from build123d import *

# Parameters (mm, degrees)
SKETCH1_W               = 40
SKETCH1_H               = 9
BOSS_EXTRUDE1_DEPTH     = 7
CUT_EXTRUDE1_DEPTH      = 5
CUT_EXTRUDE1_DEPTH_BACK = 10
SKETCH2_R               = 1
SKETCH2_R_2             = 1.4
FILLET1_R               = 10
FILLET2_R               = 0.5
SKETCH3_R               = 1.75
CUT_EXTRUDE6_DEPTH      = 3.8
SKETCH4_W               = 3.5
SKETCH4_H               = 0.5
CUT_EXTRUDE7_DEPTH      = 2.5


with BuildPart() as part:
    # Sketch1 → Boss-Extrude1 (new body)
    with BuildSketch(Plane(origin=(0, 0, 0), x_dir=(1, 0, 0), z_dir=(0, 1, 0))):
        with Locations((20, 4.5)):
            Rectangle(SKETCH1_W, SKETCH1_H)
    extrude(amount=BOSS_EXTRUDE1_DEPTH)

    # Sketch2 → Cut-Extrude1 (cut, two sides: drawn at the far end of the back side and taken through both)
    with BuildSketch(Plane(origin=(0, 7, 0), x_dir=(1, 0, 0), z_dir=(0, 1, 0)).offset(-CUT_EXTRUDE1_DEPTH_BACK)):
        with Locations(Location((8, 4, 0), (0, 0, 90))):
            Circle(SKETCH2_R)
        with Locations(Location((32, 4, 0), (0, 0, 90))):
            Circle(SKETCH2_R)
        with Locations(Location((20, 4, 0), (0, 0, 90))):
            Circle(SKETCH2_R_2)
        with BuildLine():
            ThreePointArc((21.734935157, 2.2), (20, 1.5), (18.265064843, 2.2))
            Line((18.265064843, 2.2), (11, 2.2))
            Line((11, 2.2), (16, 0.75))
            Line((16, 0.75), (24, 0.75))
            Line((24, 0.75), (29, 2.2))
            Line((29, 2.2), (21.734935157, 2.2))
        make_face()
        Polygon((13, 0.75), (8, 2.2), (3, 0.75), align=None)
        Polygon((37, 0.75), (32, 2.2), (27, 0.75), align=None)
        Polygon((0, 0.75), (5, 2.2), (0, 2.2), align=None)
        Polygon((40, 2.2), (35, 2.2), (40, 0.75), align=None)
    extrude(amount=CUT_EXTRUDE1_DEPTH + CUT_EXTRUDE1_DEPTH_BACK, mode=Mode.SUBTRACT)

    # Fillet1
    fillet1_edges = [part.edges().sort_by_distance(p)[0] for p in [
        (32, 3.5, -2.2),
        (8, 3.5, -2.2),
    ]]
    fillet(fillet1_edges, radius=FILLET1_R)

    # Fillet2
    # the kernel refuses this fillet: 0.5 mm, written as the material it adds along each edge
    with BuildSketch(Plane(origin=(24, 7, -0.75), x_dir=(0.9604291387787307, 0, -0.27852445024583705), z_dir=(0, -1, 0))) as fillet2_piece_1:
        with BuildLine():
            CenterArc((FILLET2_R * 0.142073204655, -FILLET2_R), FILLET2_R, 90, 16.172159016)
            Line((-FILLET2_R * 0.136451245591, -FILLET2_R * 0.0395708612213), (0, 0))
            Line((0, 0), (FILLET2_R * 0.142073204655, 0))
        make_face()
    extrude(amount=7)
    with BuildSketch(Plane(origin=(16, 0, -0.75), x_dir=(1, 0, 0), z_dir=(0, 1, 0))) as fillet2_piece_2:
        with BuildLine():
            CenterArc((FILLET2_R * 0.142073204655, FILLET2_R), FILLET2_R, 253.827840984, 16.172159016)
            Line((-FILLET2_R * 0.136451245591, FILLET2_R * 0.0395708612213), (0, 0))
            Line((0, 0), (FILLET2_R * 0.142073204655, 0))
        make_face()
    extrude(amount=7)
    # the kernel refuses this fillet: 0.5 mm, written as the material it takes off along each edge
    with BuildSketch(Plane(origin=(0, 7.939001537, -0.75), x_dir=(0.960429138778732, 0, -0.2785244502458324), z_dir=(0, -1, 0)), Plane(origin=(40, 7.939001537, -0.75), x_dir=(0, 0, 1), z_dir=(0, -1, 0))) as fillet2_2_piece_1:
        with BuildLine():
            CenterArc((FILLET2_R * 0.75120122935, FILLET2_R), FILLET2_R, 196.172159016, 73.827840984)
            Line((-FILLET2_R * 0.209227909429, FILLET2_R * 0.721475549754), (0, 0))
            Line((0, 0), (FILLET2_R * 0.75120122935, 0))
        make_face()
    extrude(amount=8.878003073, mode=Mode.SUBTRACT)
    with BuildSketch(Plane(origin=(0, 8.25, -2.2), x_dir=(0, 0, -1), z_dir=(0, -1, 0)), Plane(origin=(40, 8.25, -2.2), x_dir=(-1, 0, 0), z_dir=(0, -1, 0)), Plane(origin=(0, -1.25, 0), x_dir=(1, 0, 0), z_dir=(0, 1, 0))) as fillet2_2_piece_2:
        with BuildLine():
            CenterArc((FILLET2_R, FILLET2_R), FILLET2_R, 180, 90)
            Line((0, FILLET2_R), (0, 0))
            Line((0, 0), (FILLET2_R, 0))
        make_face()
    extrude(amount=9.5, mode=Mode.SUBTRACT)
    with BuildSketch(Plane(origin=(0, -1.25, -9), x_dir=(1, 0, 0), z_dir=(0, 1, 0)), Plane(origin=(40, -1.25, -9), x_dir=(0, 0, 1), z_dir=(0, 1, 0)), Plane(origin=(40, -1.25, 0), x_dir=(-1, 0, 0), z_dir=(0, 1, 0))) as fillet2_2_piece_3:
        with BuildLine():
            CenterArc((FILLET2_R, -FILLET2_R), FILLET2_R, 90, 90)
            Line((0, -FILLET2_R), (0, 0))
            Line((0, 0), (FILLET2_R, 0))
        make_face()
    extrude(amount=9.5, mode=Mode.SUBTRACT)

    # Sketch3 → Cut-Extrude6 (cut)
    with BuildSketch(Plane(origin=(0, 0, -9), x_dir=(-1, 0, 0), z_dir=(0, 0, -1))):
        with Locations((-32, 3.5)):
            Circle(SKETCH3_R)
        with Locations((-8, 3.5)):
            Circle(SKETCH3_R)
    extrude(amount=-CUT_EXTRUDE6_DEPTH, mode=Mode.SUBTRACT)

    # Sketch4 → Cut-Extrude7 (cut)
    with BuildSketch(Plane(origin=(0, 0, -5.2), x_dir=(-1, 0, 0), z_dir=(0, 0, -1))):
        with Locations((-32, 3.5)):
            Rectangle(SKETCH4_W, SKETCH4_H)
        with Locations((-8, 3.5)):
            Rectangle(SKETCH4_W, SKETCH4_H)
    extrude(amount=-CUT_EXTRUDE7_DEPTH, mode=Mode.SUBTRACT)


solid = part.part
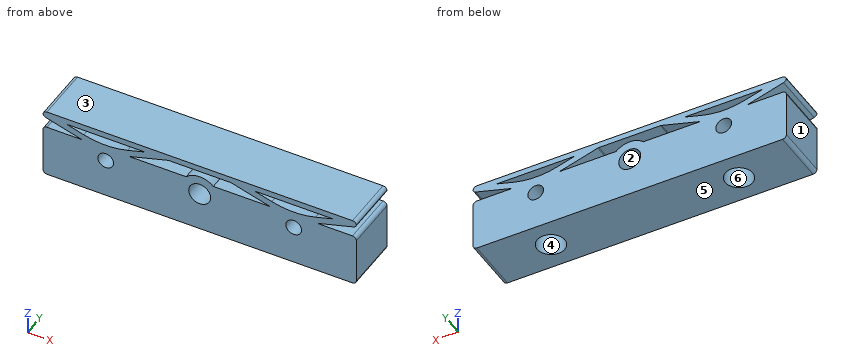
The listing builds one solid part. Answer for the finished solid, in the listing's coordinates (mm). Face numbers are marked on the shaded views. A direction names the side the tool comes from. Coordinates: 2 decimals unless noted, no trailing zeros. Write each loop counter-clockwise with the first axis right and the second up, starting at its lowest first coordinate (ties: lowest second). Pieces come first, ordered by that corner, then holes. Notation, with made-up numbers: (50.5, 62) - (106.5, 62) arc R12 ccw to (106.5, 70) - close; hole circle Ø3 at (5, 78). An arc over 180 degrees is marked (long way). Answer as CSV lines item,"result".
1. Find section B-B (x = 32). Give the vertices of the cut face in (y, z), plus the area to 3 significant figures.
Computed values:
outline,"(0, -9) - (1.75, -9) - (1.75, -5.2) - (3.25, -5.2) - (3.25, -5) - (0, -5) - close; (0, -3) - (3.25, -3) - (3.25, -2.7) - (3.75, -2.7) - (3.75, -3) - (7, -3) - (7, -1.79) - (0, -1.79) - close; (0, -0.75) - (7, -0.75) - (7, 0) - (0, 0) - close; (3.75, -5.2) - (5.25, -5.2) - (5.25, -9) - (7, -9) - (7, -5) - (3.75, -5) - close"
area,"28.2 mm²"
2. Determine the mould class of the marked faces 1, 2, 3 and 4 for opening direction X: +X half, -X half, draft (parallel to the pull), parting line (faces both ways), or undercut.
Computed values:
face 1,"-X half"
face 2,"undercut"
face 3,"draft"
face 4,"undercut"
3. Find section C-C (z = -4). Give the number of separate pieces and of enclosed holes in the cut face, plus the area to 3 significant figures.
Computed values:
separate pieces,"4"
enclosed holes,"0"
area,"231 mm²"
4. Straight lines are drawn through the part: line 1 (X direction, y = 0.85, z = -4); line 2 (Z direction, x = 22, y = 3.5); line 3 (Y direction, x = 8, z = -6.2). For each, find the intervals that lie inside material, in ascending order. Write a range as [from, to].
Computed values:
line 1,"x = [0, 7], [9, 18.6], [21.4, 31], [33, 40]"
line 2,"z = [-9, -2.2], [-0.75, 0]"
line 3,"y = [0, 1.75], [5.25, 7]"
5. Given P1, Ø1.2, axis at x = 8, z = -4, coming from the -Y side; P2, Ø0.8, axis at x = 8, y = 4.5, coming from the -Z side, each flat-ended and moving along its own axis, determine where each tip first touches the part or whether it passes through.
Computed values:
P1,"passes through"
P2,"stops at z = -5.2"
6. Find section A-A (x = 12). Give the vertices of the cut face in (y, z), plus the area to 3 significant figures.
Computed values:
outline,"(0, -9) - (7, -9) - (7, -2.2) - (0, -2.2) - close; (0, -1.91) - (7, -1.91) - (7, -1.04) - (0, -1.04) - close; (0, -0.75) - (7, -0.75) - (7, 0) - (0, 0) - close"
area,"58.9 mm²"
7. A tool of negligible diameter and unlimited length cuts with its end or side. For the marked faces 5 and 6, from which of +Z, -Z, +X, -X, +Y, -Y can it reach the whole face along a straight path? Write none if from no direction.
Computed values:
face 5,"-Z, +X, -X, +Y, -Y"
face 6,"-Z"
8. Find section D-D (x = 16.5). Give the vertices of the cut face in (y, z).
Computed values:
outline,"(0, -9) - (7, -9) - (7, -2.2) - (0, -2.2) - close; (0, -0.75) - (7, -0.75) - (7, 0) - (0, 0) - close"
